```python
from build123d import *

# Parameters (mm, degrees)
SKETCH1_W           = 105
SKETCH1_H           = 50
SKETCH1_R           = 2.25
BOSS_EXTRUDE1_DEPTH = 3.3
SKETCH2_R           = 2.65
BOSS_EXTRUDE2_DEPTH = 3.3
BOSS_EXTRUDE3_START = 3.3
SKETCH3_R           = 11
SKETCH3_R_2         = 2.65
BOSS_EXTRUDE3_DEPTH = 3.3


with BuildPart() as part:
    # Sketch1 → Boss-Extrude1 (new body)
    with BuildSketch(Plane(origin=(0, 0, 0), x_dir=(1, 0, 0), z_dir=(0, 1, 0))):
        Rectangle(SKETCH1_W, SKETCH1_H)
        with Locations(Location((-27.5, 6.5, 0), (0, 0, 270))):
            Circle(SKETCH1_R, mode=Mode.SUBTRACT)
        with Locations(Location((-27.5, -6, 0), (0, 0, 270))):
            Circle(SKETCH1_R, mode=Mode.SUBTRACT)
        with Locations(Location((27.5, -6, 0), (0, 0, 90))):
            Circle(SKETCH1_R, mode=Mode.SUBTRACT)
        with Locations(Location((27.5, 6.5, 0), (0, 0, 90))):
            Circle(SKETCH1_R, mode=Mode.SUBTRACT)
    extrude(amount=BOSS_EXTRUDE1_DEPTH)

    # Sketch2 → Boss-Extrude2 (add)
    with BuildSketch(Plane(origin=(52.5, 0, 0), x_dir=(0, 0, -1), z_dir=(1, 0, 0))):
        Polygon((25, 0), (25, 94.157864376), (10.857864376, 108.3), (-47.928932188, 108.3), (-55, 101.228932188), (-55, 80.3), (-25, 50.3), (-25, 0), align=None)
        with Locations((-45, 98.3)):
            Circle(SKETCH2_R, mode=Mode.SUBTRACT)
        with Locations((4, 98.3)):
            Circle(SKETCH2_R, mode=Mode.SUBTRACT)
    extrude(amount=BOSS_EXTRUDE2_DEPTH)

    # Sketch3 → Boss-Extrude3 (add)
    with BuildSketch(Plane.ZY.offset(52.5).offset(BOSS_EXTRUDE3_START)):
        with BuildLine():
            Line((47.928932188, 108.3), (69, 108.3))
            ThreePointArc((69, 108.3), (83, 94.3), (69, 80.3))
            Line((69, 80.3), (55, 80.3))
            Line((55, 80.3), (25, 50.3))
            Line((25, 50.3), (25, 0))
            Line((25, 0), (-25, 0))
            Line((-25, 0), (-25, 94.157864376))
            Line((-25, 94.157864376), (-10.857864376, 108.3))
            Line((-10.857864376, 108.3), (47.928932188, 108.3))
        make_face()
        with Locations((69, 94.3)):
            Circle(SKETCH3_R, mode=Mode.SUBTRACT)
        with Locations(Location((-4, 98.3, 0), (0, 0, 180))):
            Circle(SKETCH3_R_2, mode=Mode.SUBTRACT)
        with Locations(Location((45, 98.3, 0), (0, 0, 180))):
            Circle(SKETCH3_R_2, mode=Mode.SUBTRACT)
    extrude(amount=-BOSS_EXTRUDE3_DEPTH)


solid = part.part
```
Design review of the part built by this model. Coordinates are the model's own, in mm. A direction names the side the tool comes from. Coordinates: 2 decimals unless noted, no trailing zeros. Write each loop counter-clockwise with the first axis right and the second up, starting at its lowest first coordinate (ties: lowest second). Pieces come first, ordered by that corner, then holes.
1) Add section B-B (z = 6). Write out the cut boundary in (x, y), plus the area to 3 significant figures.
2) Add section A-A (x = -27.5). Write out the cut boundary in (y, z), plus the area to 3 significant figures.
3) Add section D-D (y = 23.5). Write out the cut boundary in (x, z), plus the area to 3 significant figures.
4) Mouldability with a two-part tool opening along X and no side actions: class faces 4 (the flat face through (52.5, 57, 7)), 5 (the flat face through (-55.8, 67, 6)), 6 (the cylindrical face through (54.13, 100.93, 45.34)) as +X half, -X half, draft (parallel to the pull), parting line (faces both ways), or undercut.
5) Insertion check: pin 1 (4 mm diameter, centred on y = 98.3, z = -4, fed in from +X); pin 2 (2 mm diameter, centred on x = -30.5, z = -13, fed in from +Y); pin 3 (1 mm diameter, centred on x = 54.5, y = 91, fed in from +Z); pin 4 (2.5 mm diameter, centred on x = -53.5, z = 64.5, fed in from -Y). Each pin has a flat end and moves straight along its axis. Give the tip position at first contact, or say it passes through.
6) Machinability: for faces 1 (the flat face through (-54, 108.3, 29)), 2 (the flat face through (-54, 80.3, 62)), 3 (the flat face through (54.127, 104.814, 51.415)), which of the approach directions +Z, -Z, +X, -X, +Y, -Y give a long, thin tool a straight path to every point of the face, cutting with its end or side? Answer none if there is none.
7) To check wall thickness, follow L1, parallel to X at y = 2.3, z = -6.5; L2, parallel to X at y = 56, z = 24; L3, parallel to Z at x = 27.5, y = 2.25. State the ranges of each line that lie inside material, in increasing order.
8) Add section C-C (y = 57.5). Write out the cut boundary in (x, z), plus the area to 3 significant figures.
Check result:
1. outline: (-55.8, 0) - (-29.75, 0) - (-29.75, 3.3) - (-52.5, 3.3) - (-52.5, 108.3) - (-55.8, 108.3) - close; (-25.25, 0) - (25.25, 0) - (25.25, 3.3) - (-25.25, 3.3) - close; (29.75, 0) - (55.8, 0) - (55.8, 108.3) - (52.5, 108.3) - (52.5, 3.3) - (29.75, 3.3) - close
1. area: 1,030 mm2
2. outline: (0, -25) - (3.3, -25) - (3.3, -8.75) - (0, -8.75) - close; (0, -4.25) - (3.3, -4.25) - (3.3, 3.75) - (0, 3.75) - close; (0, 8.25) - (3.3, 8.25) - (3.3, 25) - (0, 25) - close
2. area: 135 mm2
3. outline: (-55.8, -25) - (-52.5, -25) - (-52.5, 25) - (-55.8, 25) - close; (52.5, -25) - (55.8, -25) - (55.8, 25) - (52.5, 25) - close
3. area: 330 mm2
4. face 4: undercut
4. face 5: -X half
4. face 6: draft
5. pin 1: passes through
5. pin 2: stops at y = 3.3
5. pin 3: stops at z = 55
5. pin 4: stops at y = 80.3
6. face 1: +Z, -Z, +X, -X, +Y
6. face 2: +Z, +X, -X, -Y
6. face 3: +Z, +X, +Y
7. L1: x = -55.8 to -29.75, -25.25 to 25.25, 29.75 to 55.8
7. L2: x = -55.8 to -52.5, 52.5 to 55.8
7. L3: z = -25 to -8.75, -4.25 to 3.75, 8.25 to 25
8. outline: (-55.8, -25) - (-52.5, -25) - (-52.5, 32.2) - (-55.8, 32.2) - close; (52.5, -25) - (55.8, -25) - (55.8, 32.2) - (52.5, 32.2) - close
8. area: 378 mm2
